Here's how the part is built. I have some questions about the finished solid (model axes, mm). Face numbers are marked on the shaded views. A direction names the side the tool comes from. Give positions to 0.01 mm unless a question says otherwise; leave off trailing zeros. Loops run counter-clockwise (first coordinate to the right, second up) from the corner with the lowest first, then second, coordinate; pieces in that order, holes last. Notation, with made-up numbers: (50.25, 26.25) -> (95.25, 26.25) arc R29 cw to (95.25, 46.25) -> close; hole circle Ø6 at (72.25, 70). An arc over 180 degrees is marked (long way). Answer in a Markdown table with one row per item. Add a question column.
Item 1: If I drill on line 1 (Z direction, x = 23, y = 0); line 2 (Z direction, x = 9.5, y = 4); line 3 (Y direction, x = 0, z = -49.5), over which ranges is the centre line in solid material (lowest first)?
Item 2: For P1, Ø0.9, axis at x = 23.5, z = 26.5, coming from the -Y side; P2, Ø1, axis at x = 8, y = 15.5, coming from the +Z side; P3, Ø12, axis at x = -0.5, y = 19, coming from the +Z side, each with a flat end and sliding along its axis, tell me the tip position at first contact or that it passes through.
Item 3: We'd pull the mould along X, two halves only. Please class the marked faces 3, 4 and 5: released by +X, released by -X, zero draft, split by the parting line, or undercut.
Item 4: If we section it at A-A (z = 28): Write out the boundary of the cut face in (x, y), then the cut area to 3 significant figures.
Item 5: If we section it at D-D (y = -17.5): Write out the boundary of the cut face in (x, z), then the cut area to 3 significant figures.
Item 6: Which directions (+Z, -Z, +X, -X, +Y, -Y) give clear straight access to the entire face, cutting with the end or side of a thin tool? Please do the marked faces 1 and 2.
Item 7: If we section it at C-C (x = 0): Write out the boundary of the cut face in (y, z).
Item 8: If we section it at B-B (z = 45): Write out the boundary of the cut face in (x, y).
```python
from build123d import *

# Parameters (mm, degrees)
SKETCH1_R                           = 25
SKETCH1_R_2                         = 22
BOSS_EXTRUDE1_DEPTH                 = 10
SKETCH1_2_R                         = 22
BOSS_EXTRUDE2_DEPTH                 = 3
BOSS_EXTRUDE3_START                 = -7
BOSS_EXTRUDE3_DEPTH                 = 7
BOSS_EXTRUDE4_DEPTH                 = 40
CUT_EXTRUDE1_REACH                  = 74.665
CUT_EXTRUDE1_END_RADIUS             = 25
SKETCH3_R                           = 1.75
CUT_EXTRUDE1_DIRECTION_2_REACH      = 74.665
CUT_EXTRUDE1_DIRECTION_2_END_RADIUS = 25
SKETCH4_R                           = 10.25
SKETCH4_R_2                         = 8.25
BOSS_EXTRUDE5_DEPTH                 = 60
SKETCH4_2_R                         = 8.25
BOSS_EXTRUDE6_DEPTH                 = 44


with BuildPart() as part:
    # Sketch1 → Boss-Extrude1 (new body)
    with BuildSketch(Plane.XY):
        Circle(SKETCH1_R)
        Circle(SKETCH1_R_2, mode=Mode.SUBTRACT)
    extrude(amount=BOSS_EXTRUDE1_DEPTH)

    # Sketch1<2> → Boss-Extrude2 (add)
    with BuildSketch(Plane.XY):
        Circle(SKETCH1_2_R)
    extrude(amount=BOSS_EXTRUDE2_DEPTH)

    # Sketch2 → Boss-Extrude3 (add)
    with BuildSketch(Plane.XY.offset(10).offset(BOSS_EXTRUDE3_START)):
        with BuildLine():
            Line((-21.424285286, -5), (-21.424285286, 5))
            ThreePointArc((-21.424285286, 5), (-22, 0), (-21.424285286, -5))
        make_face()
        with BuildLine():
            ThreePointArc((22, 0), (21.85559741, 2.516517804), (21.424285286, 5))
            Line((21.424285286, 5), (21.424285286, -5))
            ThreePointArc((21.424285286, -5), (21.85559741, -2.516517804), (22, 0))
        make_face()
    extrude(amount=BOSS_EXTRUDE3_DEPTH)

    # Sketch2<4> → Boss-Extrude4 (add)
    with BuildSketch(Plane.XY.offset(10)):
        with BuildLine():
            Line((-21.424285286, 5), (-24.494897428, 5))
            ThreePointArc((-24.494897428, 5), (-25, 0), (-24.494897428, -5))
            Line((-24.494897428, -5), (-21.424285286, -5))
            Line((-21.424285286, -5), (-21.424285286, 5))
        make_face()
        with BuildLine():
            Line((24.494897428, 5), (21.424285286, 5))
            Line((21.424285286, 5), (21.424285286, -5))
            Line((21.424285286, -5), (24.494897428, -5))
            ThreePointArc((24.494897428, -5), (25, 0), (24.494897428, 5))
        make_face()
    extrude(amount=BOSS_EXTRUDE4_DEPTH)

    # Cut-Extrude1: up to this cylinder (the profile starts inside it)
    cut_extrude1_end = Plane(origin=(0, 0, 45), z_dir=(0, 0, -1)) * Cylinder(CUT_EXTRUDE1_END_RADIUS, 200.33, mode=Mode.PRIVATE)
    # Sketch3 → Cut-Extrude1 (cut, up to the surface)
    with BuildSketch(Plane(origin=(-21.424285286, 0, 0), x_dir=(0, 0, -1), z_dir=(1, 0, 0)), mode=Mode.PRIVATE) as cut_extrude1_sk1:
        with Locations(Location((-45, 0, 0), (0, 0, 90))):
            Circle(SKETCH3_R)
    cut_extrude1_tool1 = extrude(cut_extrude1_sk1.sketch, amount=-CUT_EXTRUDE1_REACH, mode=Mode.PRIVATE) & cut_extrude1_end
    add(cut_extrude1_tool1.solids().sort_by_distance((-21.424285, 0, 45))[0], mode=Mode.SUBTRACT)

    # Cut-Extrude1 direction 2: up to this cylinder (the profile starts inside it)
    cut_extrude1_direction_2_end = Plane(origin=(0, 0, 45), z_dir=(0, 0, -1)) * Cylinder(CUT_EXTRUDE1_DIRECTION_2_END_RADIUS, 200.33, mode=Mode.PRIVATE)
    # Sketch3 → Cut-Extrude1 direction 2 (cut, up to the surface)
    with BuildSketch(Plane(origin=(-21.424285286, 0, 0), x_dir=(0, 0, -1), z_dir=(1, 0, 0)), mode=Mode.PRIVATE) as cut_extrude1_direction_2_sk1:
        with Locations(Location((-45, 0, 0), (0, 0, 90))):
            Circle(SKETCH3_R)
    cut_extrude1_direction_2_tool1 = extrude(cut_extrude1_direction_2_sk1.sketch, amount=CUT_EXTRUDE1_DIRECTION_2_REACH, mode=Mode.PRIVATE) & cut_extrude1_direction_2_end
    add(cut_extrude1_direction_2_tool1.solids().sort_by_distance((-21.424285, 0, 45))[0], mode=Mode.SUBTRACT)

    # Sketch4 → Boss-Extrude5 (add)
    with BuildSketch(Plane(origin=(0, 0, 0), x_dir=(-1, 0, 0), z_dir=(0, 0, -1))):
        with Locations(Location((0, 0, 0), (0, 0, 180))):
            Circle(SKETCH4_R)
        Circle(SKETCH4_R_2, mode=Mode.SUBTRACT)
    extrude(amount=BOSS_EXTRUDE5_DEPTH)

    # Sketch4<2> → Boss-Extrude6 (add)
    with BuildSketch(Plane(origin=(0, 0, 0), x_dir=(-1, 0, 0), z_dir=(0, 0, -1))):
        Circle(SKETCH4_2_R)
    extrude(amount=BOSS_EXTRUDE6_DEPTH)


solid = part.part
```
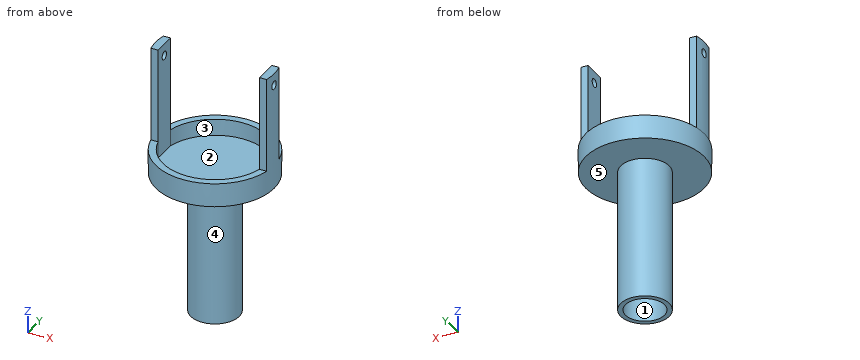
Recorded:
| question | item | result |
|---|---|---|
| 1 | line 1 | z = 0 to 43.25, 46.75 to 50 |
| 1 | line 2 | z = 0 to 3 |
| 1 | line 3 | y = -10.25 to -8.25, 8.25 to 10.25 |
| 2 | P1 | stops at y = -5 |
| 2 | P2 | stops at z = 3 |
| 2 | P3 | stops at z = 10 |
| 3 | face 3 | undercut |
| 3 | face 4 | split by the parting line |
| 3 | face 5 | zero draft |
| 4 | outline | (-24.49, -5) -> (-21.42, -5) -> (-21.42, 5) -> (-24.49, 5) arc R25 ccw to start; (21.42, -5) -> (24.49, -5) arc R25 ccw to (24.49, 5) -> (21.42, 5) -> close |
| 4 | area | 68.2 mm^2 |
| 5 | outline | (-17.85, 0) -> (17.85, 0) -> (17.85, 10) -> (13.33, 10) -> (13.33, 3) -> (-13.33, 3) -> (-13.33, 10) -> (-17.85, 10) -> close |
| 5 | area | 170 mm^2 |
| 6 | face 1 | -Z |
| 6 | face 2 | +Z |
| 7 | outline | (-25, 0) -> (-10.25, 0) -> (-10.25, -60) -> (-8.25, -60) -> (-8.25, -44) -> (8.25, -44) -> (8.25, -60) -> (10.25, -60) -> (10.25, 0) -> (25, 0) -> (25, 10) -> (22, 10) -> (22, 3) -> (-22, 3) -> (-22, 10) -> (-25, 10) -> close |
| 8 | outline | (-24.94, -1.75) arc R25 ccw to (-24.49, -5) -> (-21.42, -5) -> (-21.42, -1.75) -> close; (-24.94, 1.75) -> (-21.42, 1.75) -> (-21.42, 5) -> (-24.49, 5) arc R25 ccw to start; (21.42, -5) -> (24.49, -5) arc R25 ccw to (24.94, -1.75) -> (21.42, -1.75) -> close; (21.42, 1.75) -> (24.94, 1.75) arc R25 ccw to (24.49, 5) -> (21.42, 5) -> close |
